Work out the finished part from the listing and answer in its coordinate system (mm). Face numbers are marked on the shaded views. Give positions to 0.01 mm unless a question says otherwise; leave off trailing zeros. Loops run counter-clockwise (first coordinate to the right, second up) from the corner with the lowest first, then second, coordinate; pieces in that order, holes last. Notation, with made-up numbers: (58.25, -31.75) - (80.25, -31.75) arc R25 ccw to (80.25, -9.75) - close; hole circle Ø5 at (-33.75, 54.5). An arc over 180 degrees is marked (long way). One line per question, with ' | ' between items. Start each with the question number.
1. Section B-B (x = -1.65) is taken. Determine the outline of the cut face in (y, z), plus the area to 3 significant figures.
2. Find the intervals of material crossed by line 1 (Z direction, x = -0.8, y = 31); line 2 (X direction, y = 4, z = -0.85); line 3 (X direction, y = 2, z = 0.45), in increasing order.
3. Each of these flat-tipped pins is pushed along its axis until it touches: pin 1 (2 mm diameter, centred on x = 0, z = 0, fed in from -Y); pin 2 (2 mm diameter, centred on x = 0.5, z = -0.5, fed in from +Y). Where does it stop, or does it pass through?
4. Section A-A (y = 17.5) is taken. Determine the outline of the cut face in (x, z).
5. For a pull along Z with two mould halves and no side action, classify the marked faces 1 and 2 as released by +Z, released by -Z, zero draft, split by the parting line, or undercut.
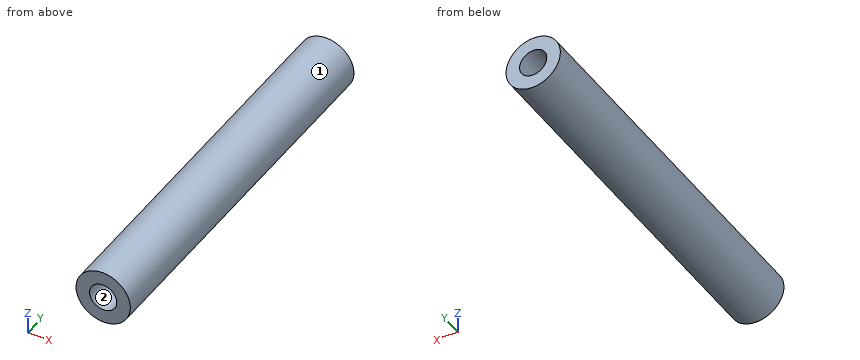
from build123d import *

# Parameters (mm, degrees)
SKETCH1_R                   = 2.5
BOSS_EXTRUDE1_DEPTH         = 34
TAP_DRILL_FOR_M3_TAP1_D     = 2.5
TAP_DRILL_FOR_M3_TAP1_DEPTH = 8
TAP_DRILL_FOR_M3_TAP1_TIP   = 0.751075774
TAP_DRILL_FOR_M3_TAP2_D     = 2.5
TAP_DRILL_FOR_M3_TAP2_DEPTH = 8
TAP_DRILL_FOR_M3_TAP2_TIP   = 0.751075774


with BuildPart() as part:
    # Sketch1 → Boss-Extrude1 (new body)
    with BuildSketch(Plane(origin=(0, 0, 0), x_dir=(1, 0, 0), z_dir=(0, 1, 0))):
        with Locations(Location((0, 0, 0), (0, 0, 270))):
            Circle(SKETCH1_R)
    extrude(amount=BOSS_EXTRUDE1_DEPTH)

    # Tap Drill for M3 Tap1
    with Locations(Plane(origin=(0, 34, 0), x_dir=(1, 0, 0), z_dir=(0, 1, 0))):
        with Locations((0, 0)):
            Hole(TAP_DRILL_FOR_M3_TAP1_D / 2, depth=TAP_DRILL_FOR_M3_TAP1_DEPTH)
            with Locations((0, 0, -(TAP_DRILL_FOR_M3_TAP1_DEPTH + TAP_DRILL_FOR_M3_TAP1_TIP / 2))):  # 118° drill point
                Cone(0, TAP_DRILL_FOR_M3_TAP1_D / 2, TAP_DRILL_FOR_M3_TAP1_TIP, mode=Mode.SUBTRACT)

    # Tap Drill for M3 Tap2
    with Locations(Plane(origin=(0, 0, 0), x_dir=(-1, 0, 0), z_dir=(0, -1, 0))):
        with Locations((0, 0)):
            Hole(TAP_DRILL_FOR_M3_TAP2_D / 2, depth=TAP_DRILL_FOR_M3_TAP2_DEPTH)
            with Locations((0, 0, -(TAP_DRILL_FOR_M3_TAP2_DEPTH + TAP_DRILL_FOR_M3_TAP2_TIP / 2))):  # 118° drill point
                Cone(0, TAP_DRILL_FOR_M3_TAP2_D / 2, TAP_DRILL_FOR_M3_TAP2_TIP, mode=Mode.SUBTRACT)


solid = part.part
Conclusion:
1) outline: (0, -1.88) - (34, -1.88) - (34, 1.88) - (0, 1.88) - close | area: 128 mm²
2) line 1: -2.37 to -0.96, 0.96 to 2.37 | line 2: -2.35 to -0.92, 0.92 to 2.35 | line 3: -2.46 to -1.17, 1.17 to 2.46
3) pin 1: y = 8.15 | pin 2: y = 34
4) outline: circle Ø5 at (0, 0)
5) face 1: split by the parting line | face 2: undercut
